For this review, take the finished solid that the model builds, in its own axes (mm). Face numbers are marked on the shaded views. A direction names the side the tool comes from. Coordinates: 2 decimals unless noted, no trailing zeros. Loops run counter-clockwise (first coordinate to the right, second up) from the corner with the lowest first, then second, coordinate; pieces in that order, holes last. Notation, with made-up numbers: (-11, -6) - (-3, -6) arc R30 cw to (-3, 18) - close; hole circle Ø4 at (45.25, 50.5). An arc over 180 degrees is marked (long way). Answer as a JSON object with one key per item and string values. Group by question number.
Item 1: We need section A-A (z = -19). Give the boundary of the cut face in (x, y), then the cut area to 3 significant figures.
Item 2: Clearance check with flat-ended pins moving along their axes: pin 1 (10.5 mm diameter, centred on x = 35.5, z = -23.5, fed in from -Y); pin 2 (4 mm diameter, centred on y = 5.5, z = 2.5, fed in from -X); pin 3 (5.5 mm diameter, centred on x = -30.5, y = 19, fed in from +Z) (3 decimals); pin 4 (6.5 mm diameter, centred on x = -14, z = 19, fed in from -Y). State where each tip first meets the part, or that it passes through.
Item 3: To check wall thickness, follow line 1 (X direction, y = 9.25, z = 0); line 2 (Z direction, x = -0.5, y = 2.5); line 3 (Z direction, x = -33, y = 19.25) (3 decimals). State the ranges of each line that lie inside material, in increasing order.
Item 4: We need section C-C (z = 0). Give the boundary of the cut face in (x, y), then the cut area to 3 significant figures.
Item 5: We need section D-D (y = 10.5). Give the boundary of the cut face in (x, z).
Item 6: Tool access review of the marked faces 1 and 2: name each direction out of +Z, -Z, +X, -X, +Y, -Y from which nothing blocks a thin tool from reaching the whole face with its end or side.
Item 7: We need section B-B (x = 9). Give the boundary of the cut face in (y, z), then the cut area to 3 significant figures.
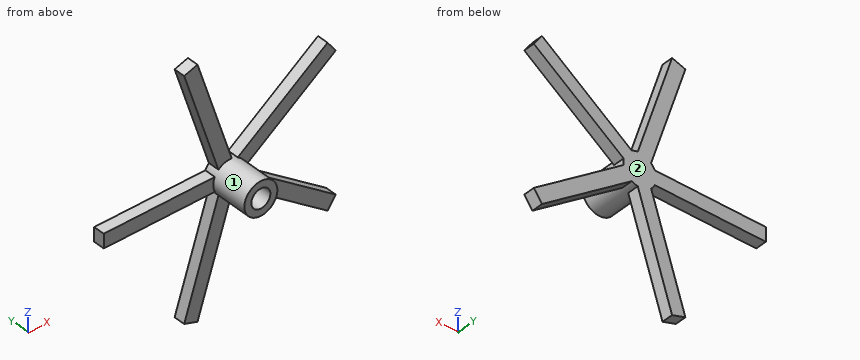
from build123d import *

# Parameters (mm, degrees)
SKETCH1_R           = 7.493
SKETCH1_R_2         = 4.318
BOSS_EXTRUDE1_DEPTH = 21.59
SKETCH2_W           = 57.15
SKETCH2_H           = 5.08
BOSS_EXTRUDE2_DEPTH = 3.175
CIRPATTERN1_COUNT   = 5


with BuildPart() as part:
    # Sketch1 → Boss-Extrude1 (new body)
    with BuildSketch(Plane(origin=(0, 0, 0), x_dir=(1, 0, 0), z_dir=(0, 1, 0))):
        with Locations(Location((0, 0, 0), (0, 0, 270))):
            Circle(SKETCH1_R)
        with Locations(Location((0, 0, 0), (0, 0, 270))):
            Circle(SKETCH1_R_2, mode=Mode.SUBTRACT)
    extrude(amount=BOSS_EXTRUDE1_DEPTH)

    # Sketch2 → Boss-Extrude2 (add, symmetric)
    with BuildSketch(Plane.XY):
        with Locations((-28.575, 19.05)):
            Rectangle(SKETCH2_W, SKETCH2_H)
    boss_extrude2 = extrude(amount=BOSS_EXTRUDE2_DEPTH, both=True)

    # CirPattern1: Boss-Extrude2 ×5 about axis
    cirpattern1_axis = Axis((0, 0, 0), (0, 1, 0))
    for i in range(1, CIRPATTERN1_COUNT):
        add(boss_extrude2.rotate(cirpattern1_axis, i * 360 / CIRPATTERN1_COUNT))


solid = part.part
Check sheet entries:
{
 "1": {"outline": "(-9.51, 16.51) - (-2.84, 16.51) - (-2.84, 21.59) - (-9.51, 21.59) - close; (20.75, 16.51) - (31.55, 16.51) - (31.55, 21.59) - (20.75, 21.59) - close", "area": "88.8 mm2"},
 "2": {"pin 1": "stops at y = 16.51", "pin 2": "stops at x = -7.48", "pin 3": "stops at z = 3.175", "pin 4": "passes through"},
 "3": {"line 1": "x = -7.49 to -4.32, 4.32 to 7.49", "line 2": "z = -7.48 to -4.29, 4.29 to 7.48", "line 3": "z = -3.175 to 3.175"},
 "4": {"outline": "(-57.15, 16.51) - (-7.49, 16.51) - (-7.49, 0) - (-4.32, 0) - (-4.32, 16.51) - (4.32, 16.51) - (4.32, 0) - (7.49, 0) - (7.49, 21.59) - (-57.15, 21.59) - close", "area": "433 mm2"},
 "5": {"outline": "circle Ø14.99 at (0, 0); hole circle Ø8.64 at (0, 0)"},
 "6": {"face 1": "-Y", "face 2": "+Z, -Z, +X, -X, +Y"},
 "7": {"outline": "(16.51, -10.46) - (21.59, -10.46) - (21.59, -2.61) - (16.51, -2.61) - close; (16.51, 2.61) - (21.59, 2.61) - (21.59, 10.46) - (16.51, 10.46) - close", "area": "79.7 mm2"}
}
